The figure shows three views and two pictorial views of one solid part (mm, origin at its lowest corner). Answer the questions. Coordinates: 2 decimals unless noted, no trailing zeros. Write each loop counter-clockwise with the first axis right and the second up, starting at its lowest first coordinate (ties: lowest second). Pieces come first, ordered by that corner, then holes. Notation, with made-up numbers: M -16,27 L 2,27 A30 cw 2,65 Z; hole C -39,-9.5 d11. An arc over 180 degrees is marked long. Write item = value, one per line. Start each with the question number.
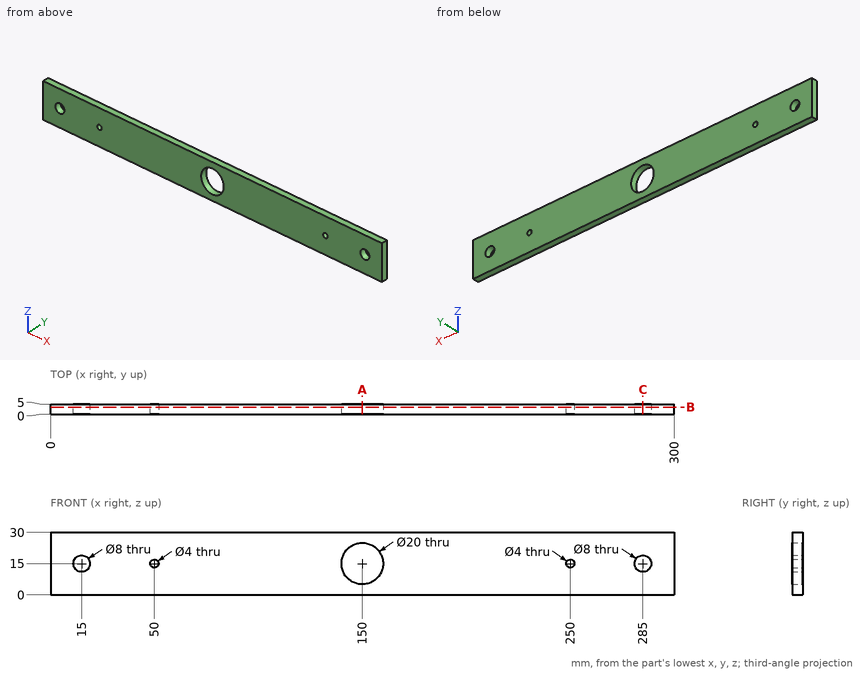
1. This flat-tipped pin is pushed along its axis until it touches: pin 1 (2.5 mm diameter, centred on x = 250, z = 15, fed in from -Y). Where does it stop, or does it pass through?
2. The part is cut by section B-B, the plane y = 3.45. Write down the section's boundary in (x, z), and give its area (3 significant figures).
3. The part is cut by section A-A, the plane x = 150. Write down the section's boundary in (y, z), and give its area (3 significant figures).
4. Straight lines are drawn through the part: L1, parallel to X at y = 3.95, z = 15; L2, parallel to Z at x = 285, y = 1.7; L3, parallel to X at y = 0.8, z = 18.5. For each, find the intervals that lie inside material, in ascending order. Write a range as [from, to].
5. The part is cut by section C-C, the plane x = 285. Write down the section's boundary in (y, z), and give its area (3 significant figures).
Solution:
q1.pin_1 = through
q2.outline = M 0,0 L 300,0 L 300,30 L 0,30 Z; hole C 15,15 d8; hole C 50,15 d4; hole C 150,15 d20; hole C 250,15 d4; hole C 285,15 d8
q2.area = 8,560 mm^2
q3.outline = M 0,0 L 5,0 L 5,5 L 0,5 Z; M 0,25 L 5,25 L 5,30 L 0,30 Z
q3.area = 50.0 mm^2
q4.L1 = [0, 11], [19, 48], [52, 140], [160, 248], [252, 281], [289, 300]
q4.L2 = [0, 11], [19, 30]
q4.L3 = [0, 13.06], [16.94, 140.63], [159.37, 283.06], [286.94, 300]
q5.outline = M 0,0 L 5,0 L 5,11 L 0,11 Z; M 0,19 L 5,19 L 5,30 L 0,30 Z
q5.area = 110 mm^2
